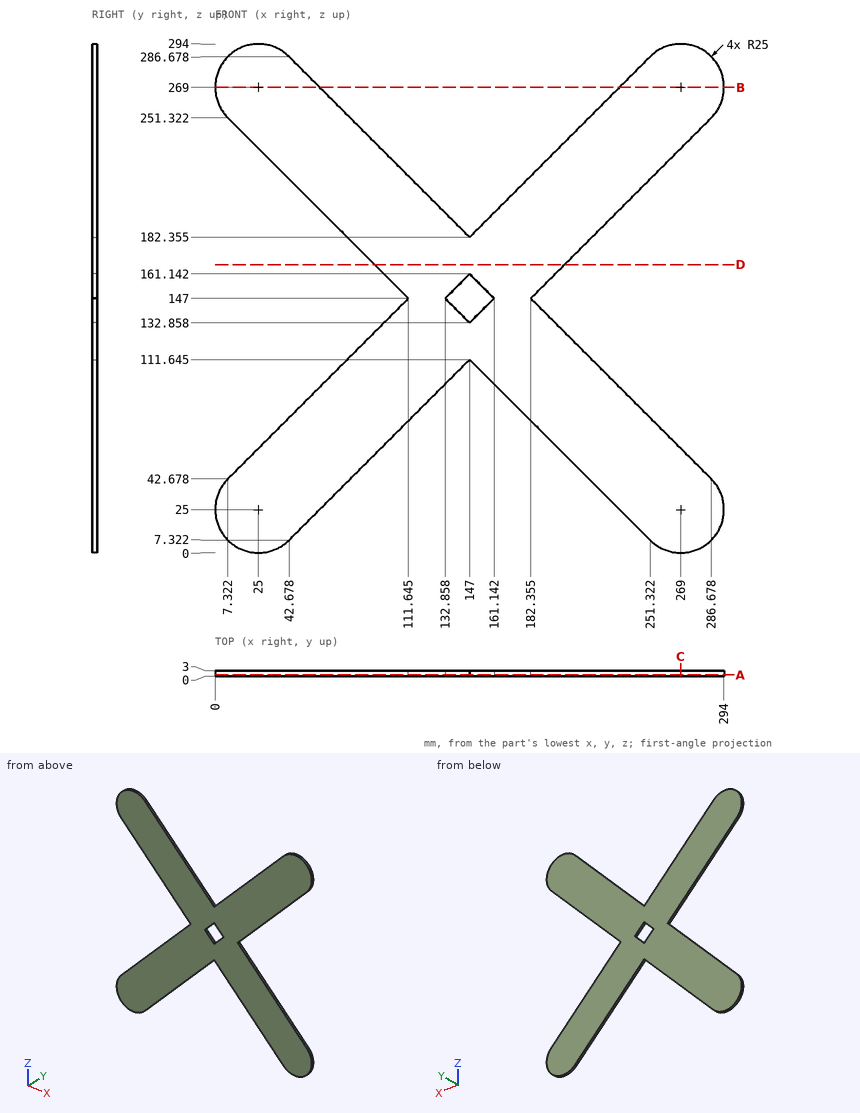
Answer from the drawing. Dimensions are ordinates in mm from the lowest x, y and z of the part. Round coordinates to 2 decimals unless told otherwise and drop trailing zeros. Loops run counter-clockwise (first coordinate to the right, second up) from the corner with the lowest first, then second, coordinate; pieces in that order, holes last. Notation, with made-up numbers: (69.5, 30.25) - (128.5, 30.25) arc R17 ccw to (128.5, 59.25) - close; hole circle Ø11 at (10, 46). An arc over 180 degrees is marked (long way). Return JSON: item names as keys, results as strings. Group by question number.
1. Each of these flat-tipped pins is pushed along its axis until it touches: P1, Ø1, axis at y = 2.5, z = 221.5, coming from the -X side (1 decimal); P2, Ø1.5, axis at y = 1.5, z = 133.5, coming from the -X side (1 decimal). Where does it stop, or does it pass through?
2. The part is cut by section A-A on y = 0.65. Determine the outline of the cut face in (x, z) (1 decimal).
3. Consider probe 1 along X at (y, z) = (2.85, 219.5) (1 decimal); probe 2 along X at (y, z) = (0.65, 68.5) (1 decimal); probe 3 along Z at (x, y) = (43, 2.8) (1 decimal). Determine where each line is inside the solid, lowest interval first.
4. The part is cut by section D-D on z = 166.5. Determine the outline of the cut face in (x, y) (1 decimal).
5. The part is cut by section B-B on z = 269. Determine the outline of the cut face in (x, y) (1 decimal), then the cut area to 3 significant figures.
6. The part is cut by section C-C on x = 269. Determine the outline of the cut face in (y, z) (1 decimal), then the cut area to 3 significant figures.
Resolved:
{
 "1": {"P1": "stops at x = 36.6", "P2": "stops at x = 97.4"},
 "2": {"outline": "(7.3, 42.7) arc R25 ccw to (42.7, 7.3) - (147, 111.6) - (251.3, 7.3) arc R25 ccw to (286.7, 42.7) - (182.4, 147) - (286.7, 251.3) arc R25 ccw to (251.3, 286.7) - (147, 182.4) - (42.7, 286.7) arc R25 ccw to (7.3, 251.3) - (111.6, 147) - close; hole (132.9, 147) - (147, 132.9) - (161.1, 147) - (147, 161.1) - close"},
 "3": {"probe 1": "x = 39.1 to 109.9, 184.1 to 254.9", "probe 2": "x = 33.1 to 103.9, 190.1 to 260.9", "probe 3": "z = 7.6 to 78.4, 215.6 to 286.4"},
 "4": {"outline": "(92.1, 0) - (201.9, 0) - (201.9, 3) - (92.1, 3) - close"},
 "5": {"outline": "(0, 0) - (60.4, 0) - (60.4, 3) - (0, 3) - close; (233.6, 0) - (294, 0) - (294, 3) - (233.6, 3) - close", "area": "362 mm²"},
 "6": {"outline": "(0, 0) - (3, 0) - (3, 60.4) - (0, 60.4) - close; (0, 233.6) - (3, 233.6) - (3, 294) - (0, 294) - close", "area": "362 mm²"}
}
